```python
from build123d import *

# Parameters (mm, degrees)
F1_DEPTH = 31.75
F3_DEPTH = 12.7
F5_DEPTH = 12.7
F7_DEPTH = 12.7


with BuildPart() as f1:
    # F0 (on Front) → F1 (new body)
    with BuildSketch(Plane.XZ):
        Polygon((-78.642312, 38.1), (-78.642312, 0), (-46.892312, 0), (-46.892312, 12.7), (-8.792312, 12.7), (-8.792312, 25.4), (-46.892312, 25.4), (-46.892312, 38.1), align=None)
    extrude(amount=F1_DEPTH)

    # F2 (on face) → F3 (cut)
    with BuildSketch(Plane(origin=(0, 0, 0), x_dir=(1, 0, 0), z_dir=(0, 0, -1))):
        Polygon((-46.892312, 31.75), (-62.767312, 31.75), (-46.892312, 0), align=None)
    extrude(amount=-F3_DEPTH, mode=Mode.SUBTRACT)

    # F4 (on face) → F5 (cut)
    with BuildSketch(Plane.XY.offset(38.1)):
        Polygon((-46.892312, 0), (-59.592312, -31.75), (-46.892312, -31.75), align=None)
    extrude(amount=-F5_DEPTH, mode=Mode.SUBTRACT)

    # F6 (on face) → F7 (cut)
    with BuildSketch(Plane(origin=(0, 0, 12.7), x_dir=(1, 0, 0), z_dir=(0, 0, -1))):
        Polygon((-8.792312, 31.75), (-21.492312, 31.75), (-8.792312, 0), align=None)
    extrude(amount=-F7_DEPTH, mode=Mode.SUBTRACT)


solid = f1.part
```
Build history of the part. All positions in model axes, mm. A direction names the side the tool comes from. Coordinates: 2 decimals unless noted, no trailing zeros. Write each loop counter-clockwise with the first axis right and the second up, starting at its lowest first coordinate (ties: lowest second). Pieces come first, ordered by that corner, then holes.
1. Band-saw the part on D-D, the plane z = 18.5. Give the cut face in (x, y).
Answer block:
outline: (-78.64, -31.75) - (-21.49, -31.75) - (-8.79, 0) - (-78.64, 0) - close
2. 3-axis set-ups, long thin cutter, end or side, ignore diameter. For faces 4 (the flat face through (-53.153, -15.653, 31.839)), 5 (the flat face through (-36, -16, 12.7)), 6 (the flat face through (-57, -31.75, 19)): which of +Z, -Z, +X, -X, +Y, -Y reach the whole face in a straight line?
Answer block:
face 4: +Z, +X, -Y
face 5: -Z, +X, -Y
face 6: +Z, -Z, +X, -X, -Y
3. Band-saw the part on A-A, the plane x = -48. Give the cut face in (y, z), and give its area (3 significant figures).
Answer block:
outline: (-31.75, 12.7) - (-2.22, 12.7) - (-2.22, 0) - (0, 0) - (0, 38.1) - (-2.77, 38.1) - (-2.77, 25.4) - (-31.75, 25.4) - close
area: 467 mm2
4. Drop flat-ended pins along their axis: pin 1 (1.5 mm diameter, centred on x = -42.5, y = -16.5, fed in from -Z); pin 2 (8 mm diameter, centred on x = -45, y = -28.5, fed in from +Z); pin 3 (2 mm diameter, centred on y = -6, z = 8.5, fed in from +X); pin 4 (4 mm diameter, centred on x = -56, y = -19.5, fed in from -Z). Give the stop position or say it passes through.
Answer block:
pin 1: stops at z = 12.7
pin 2: stops at z = 25.4
pin 3: stops at x = -49.39
pin 4: stops at z = 0
5. Drill centre lines: probe 1 along Z at (x, y) = (-22, -8.5); probe 2 along X at (y, z) = (-16, 19); probe 3 along X at (y, z) = (-2, 20.5). Where is each one in solid material? Low to high.
Answer block:
probe 1: z = 12.7 to 25.4
probe 2: x = -78.64 to -15.19
probe 3: x = -78.64 to -9.59
6. Band-saw the part on C-C, the plane z = 34.5. Give the cut face in (x, y).
Answer block:
outline: (-78.64, -31.75) - (-59.59, -31.75) - (-46.89, 0) - (-78.64, 0) - close
7. Pull direction X, two halves, no side cores. Call faces 1 (the flat face through (-54.941, -16.097, 6.261)), 2 (the flat face through (-34, -16, 25.4)), 3 (the flat face through (-78.642, -16, 19)): released by +X, released by -X, zero draft, split by the parting line, or undercut.
Answer block:
face 1: released by +X
face 2: zero draft
face 3: released by -X
8. Band-saw the part on B-B, the plane y = -6. Give the cut face in (x, z), and give its area (3 significant figures).
Answer block:
outline: (-78.64, 0) - (-49.89, 0) - (-49.89, 12.7) - (-11.19, 12.7) - (-11.19, 25.4) - (-49.29, 25.4) - (-49.29, 38.1) - (-78.64, 38.1) - close
area: 1,590 mm2
